Can you work these out from the model? Positions are in its coordinate system, mm. A direction names the side the tool comes from. Give positions to 0.01 mm unless a question says otherwise; leave off trailing zeros. Write each loop counter-clockwise with the first axis right and the second up, starting at its lowest first coordinate (ties: lowest second). Pieces come first, ordered by that corner, then holes. Notation, with made-up numbers: (-35.5, 36) -> (-27.5, 36) arc R23 ccw to (-27.5, 50) -> close; hole circle Ø4 at (32.5, 69.5). An arc over 180 degrees is marked (long way). One line per item, written item: value.
from build123d import *

# Parameters (mm, degrees)
BOSS_EXTRUDE1_DEPTH   = 60
SKETCH1_W             = 10.993820537
SKETCH1_H             = 26.396502677
BOSS_EXTRUDE1_2_DEPTH = 60
BOSS_EXTRUDE2_DEPTH   = 3
SKETCH3_W             = 21.528788888
SKETCH3_H             = 11.346253603
BOSS_EXTRUDE3_DEPTH   = 15
SKETCH4_W             = 21.528788888
SKETCH4_H             = 9.567300702
BOSS_EXTRUDE4_DEPTH   = 200
SKETCH5_W             = 51.310621716
SKETCH5_H             = 17.784956531
CUT_EXTRUDE1_DEPTH    = 200
SKETCH6_W             = 45.030110597
SKETCH6_H             = 35.891646976
CUT_EXTRUDE2_DEPTH    = 200
SKETCH7_W             = 70
SKETCH7_H             = 13
BOSS_EXTRUDE5_DEPTH   = 2
FILLET1_R             = 10
FILLET3_R             = 4
BOSS_EXTRUDE6_DEPTH   = 7


with BuildPart() as part:
    # Sketch1 → Boss-Extrude1 (new body)
    with BuildSketch(Plane.XY):
        Polygon((-19.757378597, 18.307693349), (11.507697245, 18.307693349), (11.507697245, 26.038756838), (-27.787096512, 26.038756838), (-27.787096512, 25.885892475), (-43.235049783, 10.14086318), (-35.355311996, 2.409799691), align=None)
    extrude(amount=BOSS_EXTRUDE1_DEPTH)



with BuildPart() as body_2:
    # Sketch1 → Boss-Extrude1 2 (new body)
    with BuildSketch(Plane.XY):
        with Locations((28.155491547, -37.552817793)):
            Rectangle(SKETCH1_W, SKETCH1_H)
    extrude(amount=BOSS_EXTRUDE1_2_DEPTH)


with BuildPart() as part_1:
    add(part.part)

    add(body_2.part)  # Boss-Extrude2 merges body 2
    # Sketch2 → Boss-Extrude2 (add)
    with BuildSketch(Plane.XY.offset(60)):
        Polygon((-43.235049783, 10.14086318), (-27.787096512, 26.038756838), (11.507697245, 26.038756838), (33.652401815, -24.354566454), (33.652401815, -50.751069131), (22.658581278, -50.751069131), (-35.355311996, 2.409799691), align=None)
    extrude(amount=BOSS_EXTRUDE2_DEPTH)

    # Sketch3 → Boss-Extrude3 (add)
    with BuildSketch(Plane.XY.offset(63)):
        with Locations((-2.754816927, 13.64397724)):
            Rectangle(SKETCH3_W, SKETCH3_H)
    extrude(amount=BOSS_EXTRUDE3_DEPTH)

    # Sketch4 → Boss-Extrude4 (add)
    with BuildSketch(Plane.XZ.offset(-7.970850439)):
        with Locations((-2.754816927, 73.216349649)):
            Rectangle(SKETCH4_W, SKETCH4_H)
    extrude(amount=BOSS_EXTRUDE4_DEPTH)

    # Sketch5 → Cut-Extrude1 (cut)
    with BuildSketch(Plane.ZY.offset(-22.658581278)):
        with Locations((30.574482512, -37.306256307)):
            Rectangle(SKETCH5_W, SKETCH5_H)
    extrude(amount=-CUT_EXTRUDE1_DEPTH, mode=Mode.SUBTRACT)

    # Sketch6 → Cut-Extrude2 (cut)
    with BuildSketch(Plane(origin=(0, 26.038756838, 0), x_dir=(1, 0, 0), z_dir=(0, 1, 0))):
        with Locations((-15.916410132, -24.110147888)):
            Rectangle(SKETCH6_W, SKETCH6_H)
    extrude(amount=-CUT_EXTRUDE2_DEPTH, mode=Mode.SUBTRACT)

    # Sketch7 → Boss-Extrude5 (add)
    with BuildSketch(Plane.XZ.offset(192.029149561)):
        with Locations((-2.644159555, 71.5)):
            Rectangle(SKETCH7_W, SKETCH7_H)
    extrude(amount=BOSS_EXTRUDE5_DEPTH)

    # Fillet1
    fillet1_edges = [part_1.edges().sort_by_distance(p)[0] for p in [
        (-13.519211371, -192.029149561, 73.216349649),
        (8.009577517, -192.029149561, 73.216349649),
    ]]
    fillet(fillet1_edges, radius=FILLET1_R)

    # Fillet3
    # the kernel refuses this fillet: 4 mm, written as the material it adds along each edge
    with BuildSketch(Plane(origin=(8.009577517, 7.970850439, 63), x_dir=(0, 0, 1), z_dir=(-1, 0, 0)), Plane(origin=(8.009577517, 7.970850439, 68.432699298), x_dir=(0, -1, 0), z_dir=(-1, 0, 0))) as fillet3_piece_1:
        with BuildLine():
            CenterArc((FILLET3_R, -FILLET3_R), FILLET3_R, 90, 90)
            Line((0, -FILLET3_R), (0, 0))
            Line((0, 0), (FILLET3_R, 0))
        make_face()
    extrude(amount=21.528788888)

    # Sketch8 → Boss-Extrude6 (add)
    with BuildSketch(Plane(origin=(0, 0, 68.432699298), x_dir=(-1, 0, 0), z_dir=(0, 0, -1))):
        Polygon((10.906624275, -19.993686913), (-1.270597079, -31.152249638), (-5.600185218, -26.427415943), (6.577036136, -15.268853218), align=None)
    extrude(amount=BOSS_EXTRUDE6_DEPTH)


solid = part_1.part
1) For faces 4 (the face through (-0.4, -20.93, 65.75)), 5 (the face through (-27.666, 10.247, 50.902)), 6 (the face through (-2.6, 6.33, 63.77)), 7 (the face through (11.508, 22, 30)), 8 (the face through (-38.431, 10, 24)), which set-ups out of +Z, -Z, +X, -X, +Y, -Y let a thin tool reach every point of the face, with its end or its side?
Answer list:
face 4: +X
face 5: -Z, +X, -Y
face 6: +X, -X
face 7: -Z, +X, +Y, -Y
face 8: +X, +Y, -Y
2) Will these pins go through, and if not, where does the flat tip stop? pin 1 (4 mm diameter, centred on y = -3, z = 70, fed in from -X); pin 2 (1.5 mm diameter, centred on x = -14.5, z = 67, fed in from +Y); pin 3 (12 mm diameter, centred on x = 29.5, z = 17.5, fed in from -Y).
Answer list:
pin 1: stops at x = -13.52
pin 2: stops at y = -192.03
pin 3: stops at y = -50.75
3) We'd pull the mould along Y, two halves only. Please class faces 1 (the face through (-8.712, -17.598, 65.754)), 2 (the face through (22.659, -47, 30)), 3 (the face through (11.02, -189.18, 73.28)): released by +Y, released by -Y, zero draft, split by the parting line, or undercut.
Answer list:
face 1: undercut
face 2: zero draft
face 3: released by +Y
4) I need wall thicknesses on L1, parallel to Y at x = 7.5, z = 31; L2, parallel to Z at x = -2.5, y = -22; L3, parallel to X at y = -16.5, z = 71. Which ranges of each line are inside material? Lowest first, please.
Answer list:
L1: y = 18.31 to 26.04
L2: z = 60 to 78
L3: x = -13.52 to 8.01
5) If we section it at A-A (z = 32): Write out the boundary of the cut face in (x, y), and give its area (3 significant figures).
Answer list:
outline: (-43.24, 10.14) -> (-38.43, 5.43) -> (-38.43, 15.04) -> close; (6.6, 18.31) -> (11.51, 18.31) -> (11.51, 26.04) -> (6.6, 26.04) -> close; (22.66, -50.75) -> (33.65, -50.75) -> (33.65, -46.2) -> (22.66, -46.2) -> close; (22.66, -28.41) -> (33.65, -28.41) -> (33.65, -24.35) -> (22.66, -24.35) -> close
area: 156 mm^2
6) If we section it at B-B (z = 48): Write out the boundary of the cut face in (x, y).
Answer list:
outline: (-43.24, 10.14) -> (-35.36, 2.41) -> (-19.76, 18.31) -> (11.51, 18.31) -> (11.51, 26.04) -> (-27.79, 26.04) -> (-27.79, 25.89) -> close; (22.66, -50.75) -> (33.65, -50.75) -> (33.65, -46.2) -> (22.66, -46.2) -> close; (22.66, -28.41) -> (33.65, -28.41) -> (33.65, -24.35) -> (22.66, -24.35) -> close
7) If we section it at C-C (x = -2): Write out the boundary of the cut face in (y, z), and give its area (3 significant figures).
Answer list:
outline: (-194.03, 65) -> (-192.03, 65) -> (-192.03, 68.43) -> (-28.16, 68.43) -> (-28.16, 60) -> (18.31, 60) -> (18.31, 42.06) -> (26.04, 42.06) -> (26.04, 63) -> (19.32, 63) -> (19.32, 78) -> (-194.03, 78) -> close; (18.31, 0) -> (26.04, 0) -> (26.04, 6.16) -> (18.31, 6.16) -> close; hole (-19.46, 63) -> (3.97, 63) arc R4 ccw to (7.76, 65.72) arc R4 ccw to (3.97, 68.43) -> (-19.46, 68.43) -> close
area: 2,510 mm^2
8) If we section it at D-D (x = -33): Write out the boundary of the cut face in (y, z), and give its area (3 significant figures).
Answer list:
outline: (-194.03, 65) -> (-192.03, 65) -> (-192.03, 78) -> (-194.03, 78) -> close; (0.25, 60) -> (4.81, 60) -> (4.81, 42.06) -> (20.57, 42.06) -> (20.57, 60) -> (20.67, 60) -> (20.67, 63) -> (0.25, 63) -> close; (4.81, 0) -> (20.57, 0) -> (20.57, 6.16) -> (4.81, 6.16) -> close
area: 467 mm^2
